Geometry: final body of the model. Coordinates: model frame, mm. A direction names the side the tool comes from. Give positions to 0.01 mm unless a question says otherwise; leave off trailing zeros. Write each loop counter-clockwise with the first axis right and the second up, starting at its lowest first coordinate (ties: lowest second). Pieces come first, ordered by that corner, then holes.
```python
from build123d import *

# Parameters (mm, degrees)
SKETCH1_W           = 13
SKETCH1_H           = 16
SKETCH1_R           = 2.5
BOSS_EXTRUDE1_DEPTH = 2
FILLET1_R           = 5
SKETCH2_W           = 13
SKETCH2_H           = 2
BOSS_EXTRUDE2_DEPTH = 16
FILLET2_R           = 5
SKETCH3_R           = 2.5
CUT_EXTRUDE1_DEPTH  = 16


with BuildPart() as part:
    # Sketch1 → Boss-Extrude1 (new body)
    with BuildSketch(Plane.XY):
        Rectangle(SKETCH1_W, SKETCH1_H)
        with Locations((0, 2)):
            Circle(SKETCH1_R, mode=Mode.SUBTRACT)
    extrude(amount=BOSS_EXTRUDE1_DEPTH)

    # Fillet1
    fillet1_edges = [part.edges().sort_by_distance(p)[0] for p in [
        (-6.5, 8, 1),
        (6.5, 8, 1),
    ]]
    fillet(fillet1_edges, radius=FILLET1_R)

    # Sketch2 → Boss-Extrude2 (add)
    with BuildSketch(Plane.XY.offset(2)):
        with Locations((0, -7)):
            Rectangle(SKETCH2_W, SKETCH2_H)
    extrude(amount=BOSS_EXTRUDE2_DEPTH)

    # Fillet2
    fillet2_edges = [part.edges().sort_by_distance(p)[0] for p in [
        (-6.5, -7, 18),
        (6.5, -7, 18),
    ]]
    fillet(fillet2_edges, radius=FILLET2_R)

    # Sketch3 → Cut-Extrude1 (cut)
    with BuildSketch(Plane(origin=(0, -6, 0), x_dir=(1, 0, 0), z_dir=(0, 1, 0))):
        with Locations((0, -10)):
            Circle(SKETCH3_R)
    extrude(amount=-CUT_EXTRUDE1_DEPTH, mode=Mode.SUBTRACT)


solid = part.part
```
Item 1: Pull-direction query (X, two-part tool) for faces 3 (the face through (-0.54, -0.44, 0.99)), 4 (the face through (5.07, -6.99, 16.5)), 5 (the face through (0, -2, 0)); classes: +X half, -X half, draft (parallel to the pull), parting line (faces both ways), or undercut.
Found:
face 3: undercut
face 4: +X half
face 5: draft
Item 2: Reachability of faces 1 (the face through (3, -6, 10)), 2 (the face through (-6.5, -6.2, 5)) from +Z, -Z, +X, -X, +Y, -Y: full face, straight path, thin tool, end or side. Return the list, or none.
Found:
face 1: +Z, +X, -X, +Y
face 2: +Z, -Z, -X, +Y, -Y
Item 3: Line query: L1, parallel to Y at x = 0, z = 1.5; L2, parallel to X at y = -6.9, z = 10; L3, parallel to Z at x = 0, y = -7.1. Output: solid intervals per line, ascending.
Found:
L1: y = -8 to -0.5, 4.5 to 8
L2: x = -6.5 to -2.5, 2.5 to 6.5
L3: z = 0 to 7.5, 12.5 to 18
Item 4: Section B-B, the plane x = 0. Return the cut outline in (y, z), plus the area to 3 significant figures.
Found:
outline: (-8, 0) - (-0.5, 0) - (-0.5, 2) - (-6, 2) - (-6, 7.5) - (-8, 7.5) - close; (-8, 12.5) - (-6, 12.5) - (-6, 18) - (-8, 18) - close; (4.5, 0) - (8, 0) - (8, 2) - (4.5, 2) - close
area: 44.0 mm2
Item 5: Section A-A, the plane z = 10. Return the cut outline in (x, y).
Found:
outline: (-6.5, -8) - (-2.5, -8) - (-2.5, -6) - (-6.5, -6) - close; (2.5, -8) - (6.5, -8) - (6.5, -6) - (2.5, -6) - close
Item 6: Section D-D, the plane y = -1.25. Return the cut outline in (x, z).
Found:
outline: (-6.5, 0) - (6.5, 0) - (6.5, 2) - (-6.5, 2) - close
Item 7: Pin query (flat end, axial travel): pin 1 Ø6.5 at (x, y) = (2.5, -1.5) entering from +Z; pin 2 Ø4 at (x, z) = (5, 14.5) entering from +Y; pin 3 Ø1 at (y, z) = (6, 2) entering from +X; pin 4 Ø4.5 at (x, y) = (0, 2) entering from -Z. Return the tip coordinate at first contact, or that it passes through.
Found:
pin 1: stops at z = 2
pin 2: stops at y = -6
pin 3: stops at x = 5.83
pin 4: passes through
Item 8: Section C-C, the plane y = 2. Return the cut outline in (x, z).
Found:
outline: (-6.5, 0) - (-2.5, 0) - (-2.5, 2) - (-6.5, 2) - close; (2.5, 0) - (6.5, 0) - (6.5, 2) - (2.5, 2) - close
